Can you work these out from the drawing? Everything is in mm from the part's minimum corner. A direction names the side the tool comes from. Round coordinates to 2 decimals unless told otherwise and drop trailing zeros. Write each loop counter-clockwise with the first axis right and the second up, starting at its lowest first coordinate (ties: lowest second). Pieces come first, ordered by that corner, then holes. Notation, with made-up numbers: (59, 42.5) -> (96, 42.5) arc R16 ccw to (96, 62.5) -> close; hole circle Ø3 at (-35, -9.75). An arc over 180 degrees is marked (long way). One line per question, with ' | ' between items. Start each with the question number.
1. If I drill on line 1 along X through (y, z) = (14.8, 4); line 2 along Y through (x, z) = (3.5, 1.75); line 3 along Z through (x, y) = (38, 6), over which ranges is the centre line in solid material (lowest first)? Write a range as [from, to].
2. For the marked faces 1 and 2, which set-ups out of +Z, -Z, +X, -X, +Y, -Y let a thin tool reach every point of the face, with its end or its side?
3. Imagine slicing it at B-B, the plane z = 1. List the corners of the cut face in (x, y) for me, and give its area (3 significant figures).
4. Imagine slicing it at C-C, the plane y = 6. List the corners of the cut face in (x, z) for me.
5. Imagine slicing it at A-A, the plane x = 36. List the corners of the cut face in (y, z) for me.
6. For pin 1 Ø5 at (y, z) = (11.5, 8.5) entering from -X; pin 2 Ø3 at (x, z) = (34.5, 1.5) entering from -Y; pin 3 Ø6 at (x, y) = (6.5, 9) entering from -Z; pin 4 Ø2 at (x, y) = (29, 6) entering from -Z, each with a flat end and sliding along its axis, tell me the tip position at first contact or that it passes through.
7. Imagine slicing it at D-D, the plane x = 2. List the corners of the cut face in (y, z) for me.
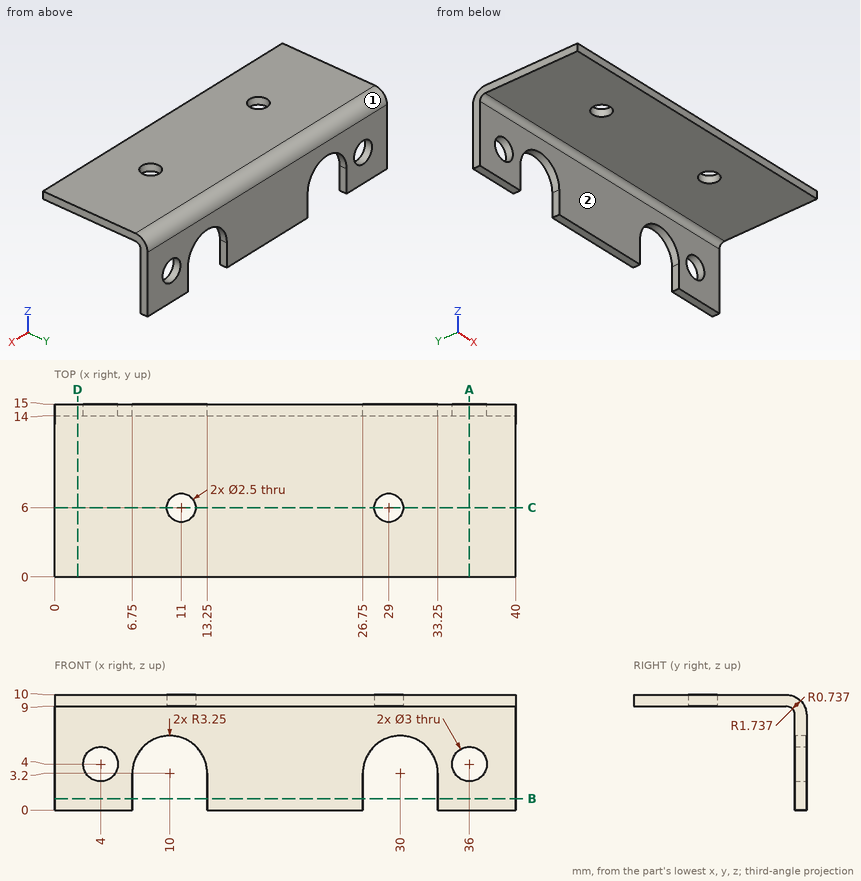
Geometry results:
1) line 1: x = [0, 2.5], [5.5, 6.85], [13.15, 26.85], [33.15, 34.5], [37.5, 40] | line 2: y = [14, 15] | line 3: z = [9, 10]
2) face 1: +Z, +X, -X, +Y | face 2: -Z, +X, -X, -Y
3) outline: (0, 14) -> (6.75, 14) -> (6.75, 15) -> (0, 15) -> close; (13.25, 14) -> (26.75, 14) -> (26.75, 15) -> (13.25, 15) -> close; (33.25, 14) -> (40, 14) -> (40, 15) -> (33.25, 15) -> close | area: 27.0 mm2
4) outline: (0, 9) -> (9.75, 9) -> (9.75, 10) -> (0, 10) -> close; (12.25, 9) -> (27.75, 9) -> (27.75, 10) -> (12.25, 10) -> close; (30.25, 9) -> (40, 9) -> (40, 10) -> (30.25, 10) -> close
5) outline: (0, 9) -> (13.26, 9) arc R0.74 cw to (14, 8.26) -> (14, 5.5) -> (15, 5.5) -> (15, 8.26) arc R1.74 ccw to (13.26, 10) -> (0, 10) -> close; (14, 0) -> (15, 0) -> (15, 2.5) -> (14, 2.5) -> close
6) pin 1: stops at x = 0 | pin 2: stops at y = 14 | pin 3: stops at z = 9 | pin 4: passes through
7) outline: (0, 9) -> (13.26, 9) arc R0.74 cw to (14, 8.26) -> (14, 0) -> (15, 0) -> (15, 8.26) arc R1.74 ccw to (13.26, 10) -> (0, 10) -> close
